The model under review builds one solid part; all positions refer to its coordinate system, in mm. Face numbers are marked on the shaded views. A direction names the side the tool comes from. Coordinates: 2 decimals unless noted, no trailing zeros. Write each loop counter-clockwise with the first axis right and the second up, starting at its lowest first coordinate (ties: lowest second). Pieces come first, ordered by that corner, then holes. Notation, with made-up numbers: (74, 0.5) -> (97, 0.5) arc R31 ccw to (97, 31.5) -> close; hole circle Ø9 at (81.5, 25.25). An arc over 180 degrees is marked (long way). Write each question's results on one line, items separated by ' | '.
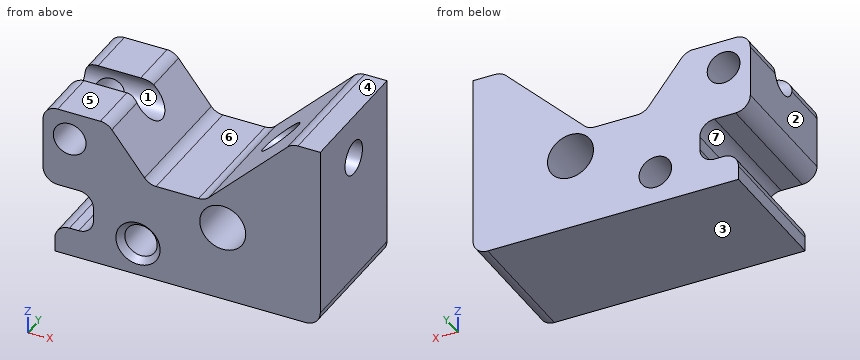
```python
from build123d import *

# Parameters (mm, degrees)
F0_R       = 7.0158249189
F0_R_2     = 7.6708
F0_R_3     = 9.9404801973
F0_R_4     = 7.0825554901
F1_DEPTH   = 55.88
F2_R       = 7.297507907
F1_FACE1_W = 55.88
F1_FACE1_H = 22.1268048838
F3_DEPTH   = 119.8785358498
F4_SIZE    = 2.54


with BuildPart() as f1:
    # F0 (on Front) → F1 (new body)
    with BuildSketch(Plane.XZ):
        with BuildLine():
            Line((-30.753318463, 45.9163933992), (-49.1895893753, 45.9163933992))
            ThreePointArc((-49.1895893753, 45.9163933992), (-53.6797174358, 44.0565214598), (-55.5395893753, 39.5663933992))
            Line((-55.5395893753, 39.5663933992), (-55.5395893753, 17.4395885155))
            ThreePointArc((-55.5395893753, 17.4395885155), (-53.6797174358, 12.9494604549), (-49.1895893753, 11.0895885155))
            Line((-49.1895893753, 11.0895885155), (-40.0770088494, 11.0895885155))
            ThreePointArc((-40.0770088494, 11.0895885155), (-35.5868807888, 9.229716576), (-33.7270088494, 4.7395885155))
            Line((-33.7270088494, 4.7395885155), (-33.7270088494, -1.0736080982))
            ThreePointArc((-33.7270088494, -1.0736080982), (-35.5868807888, -5.5637361587), (-40.0770088494, -7.4236080982))
            Line((-40.0770088494, -7.4236080982), (-44.0572159529, -7.4236080982))
            ThreePointArc((-44.0572159529, -7.4236080982), (-48.5473440134, -9.2834800376), (-50.4072159529, -13.7736080982))
            Line((-50.4072159529, -13.7736080982), (-50.4072159529, -19.8879390955))
            Line((-50.4072159529, -19.8879390955), (57.9879464746, -19.8879390955))
            ThreePointArc((57.9879464746, -19.8879390955), (62.4780745351, -18.028067156), (64.3379464746, -13.5379390955))
            Line((64.3379464746, -13.5379390955), (64.3379464746, 60.5803094804))
            Line((64.3379464746, 60.5803094804), (54.6690416703, 60.5803094804))
            ThreePointArc((54.6690416703, 60.5803094804), (52.2533179297, 60.1028539723), (50.2008699704, 58.742287058))
            Line((50.2008699704, 58.742287058), (16.1533638011, 25.0253412392))
            ThreePointArc((16.1533638011, 25.0253412392), (14.1009158419, 23.6647743249), (11.6851921012, 23.1873188168))
            Line((11.6851921012, 23.1873188168), (-6.639673132, 23.1873188168))
            ThreePointArc((-6.639673132, 23.1873188168), (-9.4073756693, 23.8222227839), (-11.6216214126, 25.5999730955))
            Line((-11.6216214126, 25.5999730955), (-25.7713701823, 43.5037391206))
            ThreePointArc((-25.7713701823, 43.5037391206), (-27.9856159257, 45.2814894321), (-30.753318463, 45.9163933992))
        make_face()
        with Locations((-14.4806178287, -5.590618588)):
            Circle(F0_R, mode=Mode.SUBTRACT)
        with Locations((48.0243302882, -7.7902064659)):
            Circle(F0_R_2, mode=Mode.SUBTRACT)
        with Locations((22.1791788936, 12.9225775599)):
            Circle(F0_R_3, mode=Mode.SUBTRACT)
        with Locations((-43.9917519689, 33.6353629827)):
            Circle(F0_R_4, mode=Mode.SUBTRACT)
        with Locations((48.0243302882, -7.7902064659)):
            Circle(F0_R_2)
    extrude(amount=F1_DEPTH)

    # F2 (on face) + F1_face1 (on face) → F3 (cut, through all)
    with BuildSketch(Plane.YZ.offset(64.3379464746)):
        with Locations((-27.8614442796, 41.5172167122)):
            Circle(F2_R)
    with BuildSketch(Plane(origin=(-55.5395893753, -27.94, 28.5029909573), x_dir=(0, -1, 0), z_dir=(-1, 0, 0))):
        Rectangle(F1_FACE1_W, F1_FACE1_H)
    extrude(amount=-F3_DEPTH, dir=(1, 0, 0), mode=Mode.SUBTRACT)

    # F4
    f4_edges = [f1.edges().sort_by_distance(p)[0] for p in [
        (-21.496443, -55.88, -5.590619),
    ]]
    chamfer(f4_edges, length=F4_SIZE)


solid = f1.part
```
Q1. Add section D-D (x = 9). Write out the cut boundary in (y, z), plus the area to 3 significant figures.
Solution:
outline: (-55.88, -19.89) -> (0, -19.89) -> (0, 23.19) -> (-55.88, 23.19) -> close | area: 2,410 mm²
Q2. Clearance check with flat-ended pins moving along their axes: P1, Ø11.5, axis at y = -27.86, z = 41.52, coming from the -X side; P2, Ø2, axis at x = -42.5, y = -31.5, coming from the +Z side; P3, Ø3, axis at y = -18, z = 2, coming from the -X side; P4, Ø20, axis at x = -2, y = -30, coming from the +Z side. State where each tip first meets the part, or that it passes through.
Solution:
P1: through | P2: z = 27.01 | P3: x = -33.73 | P4: z = 26.08
Q3. Add section C-C (y = -17.5). Write out the cut boundary in (x, z).
Solution:
outline: (-55.54, 17.44) arc R6.35 ccw to (-49.19, 11.09) -> (-40.08, 11.09) arc R6.35 cw to (-33.73, 4.74) -> (-33.73, -1.07) arc R6.35 cw to (-40.08, -7.42) -> (-44.06, -7.42) arc R6.35 ccw to (-50.41, -13.77) -> (-50.41, -19.89) -> (57.99, -19.89) arc R6.35 ccw to (64.34, -13.54) -> (64.34, 60.58) -> (54.67, 60.58) arc R6.35 ccw to (50.2, 58.74) -> (16.15, 25.03) arc R6.35 cw to (11.69, 23.19) -> (-6.64, 23.19) arc R6.35 cw to (-11.62, 25.6) -> (-25.77, 43.5) arc R6.35 ccw to (-30.75, 45.92) -> (-49.19, 45.92) arc R6.35 ccw to (-55.54, 39.57) -> close; hole circle Ø14.17 at (-43.99, 33.64); hole circle Ø14.03 at (-14.48, -5.59); hole circle Ø19.88 at (22.18, 12.92)
Q4. Add section B-B (x = 27). Write out the cut boundary in (y, z), plus the area to 3 significant figures.
Solution:
outline: (-55.88, -19.89) -> (0, -19.89) -> (0, 4.23) -> (-55.88, 4.23) -> close; (-55.88, 21.62) -> (0, 21.62) -> (0, 35.77) -> (-23.37, 35.77) arc R7.3 cw to (-32.35, 35.77) -> (-55.88, 35.77) -> close | area: 2,130 mm²
Q5. Add section A-A (y = -26). Write out the cut boundary in (x, z).
Solution:
outline: (-55.54, 17.44) arc R6.35 ccw to (-49.19, 11.09) -> (-40.08, 11.09) arc R6.35 cw to (-33.73, 4.74) -> (-33.73, -1.07) arc R6.35 cw to (-40.08, -7.42) -> (-44.06, -7.42) arc R6.35 ccw to (-50.41, -13.77) -> (-50.41, -19.89) -> (57.99, -19.89) arc R6.35 ccw to (64.34, -13.54) -> (64.34, 34.46) -> (25.68, 34.46) -> (16.15, 25.03) arc R6.35 cw to (11.69, 23.19) -> (-6.64, 23.19) arc R6.35 cw to (-11.62, 25.6) -> (-18.62, 34.46) -> (-36.96, 34.46) arc R7.08 cw (long way) to (-51.03, 34.46) -> (-55.54, 34.46) -> close; (39.93, 48.57) -> (64.34, 48.57) -> (64.34, 60.58) -> (54.67, 60.58) arc R6.35 ccw to (50.2, 58.74) -> close; hole circle Ø14.03 at (-14.48, -5.59); hole circle Ø19.88 at (22.18, 12.92)
Q6. Draft analysis for pull direction Z (two halves, no side actions). For the marked faces 1, 2, 3 and 4, state which applies: pulls with the +Z half, pulls with the -Z half, needs draft (parallel to the pull), parting line crosses it, or undercut.
Solution:
face 1: undercut | face 2: needs draft | face 3: pulls with the -Z half | face 4: pulls with the +Z half
Q7. For line 1 (X direction, y = -40, z = 29); line 2 (X direction, y = -6, z = 29.5); line 3 (Y direction, x = -28.5, z = 37.5), list the stretches that pass through material, from the lowest coordinate up. Write a range as from..to.
Solution:
line 1: -55.54..-49.35, -38.64..-14.31, 20.17..64.34 | line 2: -55.54..-49.74, -38.24..-14.7, 20.67..64.34 | line 3: -55.88..-33.95, -21.77..0
Q8. Machinability: for the marked faces 5, 6 and 7, which of the approach directions +Z, -Z, +X, -X, +Y, -Y give a long, thin tool a straight path to every point of the face, cutting with its end or side? Answer none if there is none.
Solution:
face 5: +Z, -X, +Y, -Y | face 6: +Z, +Y, -Y | face 7: -X, +Y, -Y
